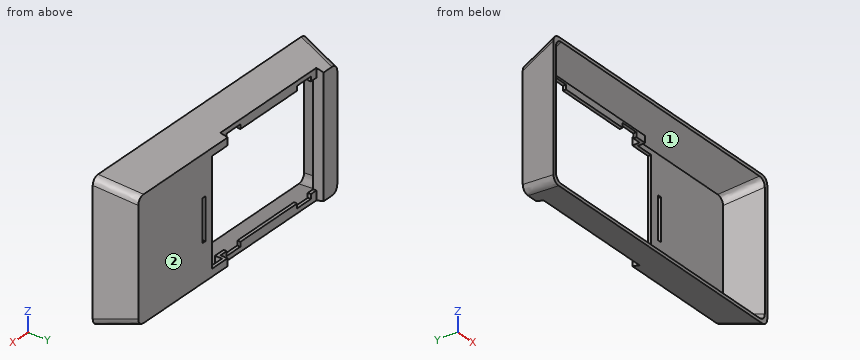
```python
from build123d import *

# Parameters (mm, degrees)
CUT_EXTRUDE1_REACH             = 225.719
SKETCH4_W                      = 175
SKETCH4_H                      = 10
CUT_EXTRUDE1_DIRECTION_2_REACH = 225.719
SHELL1_T                       = -4.4
CUT_EXTRUDE2_DEPTH             = 224.718573366
FILLET1_R                      = 10
SKETCH7_W                      = 5.5
SKETCH7_H                      = 58
CUT_EXTRUDE4_DEPTH             = 10


with BuildPart() as part:
    # Sketch2 → Loft1 section 0
    with BuildSketch(Plane(origin=(0, 0, 0), x_dir=(1, 0, 0), z_dir=(0, 1, 0))):
        with BuildLine():
            Line((-195, 96), (195, 96))
            Line((195, 96), (195, -96))
            Line((195, -96), (-195, -96))
            Line((-195, -96), (-195, 96))
        make_face()
    # Sketch3 → Loft1 section 1
    with BuildSketch(Plane(origin=(0, 53, 0), x_dir=(1, 0, 0), z_dir=(0, 1, 0))):
        with BuildLine():
            Line((-181.5, 83), (181.5, 83))
            Line((181.5, 83), (181.5, -83))
            Line((181.5, -83), (-181.5, -83))
            Line((-181.5, -83), (-181.5, 83))
        make_face()
    loft()

    # Cut-Extrude1: up to this plane
    cut_extrude1_end = Plane(origin=(0, 22.210879785, -90.552048355), z_dir=(0, -0.23822152779764819, 0.9712108440981054))
    # Sketch4 → Cut-Extrude1 (cut, up to the surface)
    with BuildSketch(Plane.XY, mode=Mode.PRIVATE) as cut_extrude1_sk1:
        with Locations((-69, 48)):
            Rectangle(SKETCH4_W, SKETCH4_H)
    cut_extrude1_tool1 = split(extrude(cut_extrude1_sk1.sketch, amount=-CUT_EXTRUDE1_REACH, mode=Mode.PRIVATE), bisect_by=cut_extrude1_end, keep=Keep.BOTH, mode=Mode.PRIVATE)
    add(cut_extrude1_tool1.solids().sort_by_distance((-69, 48, 0))[0], mode=Mode.SUBTRACT)

    # Cut-Extrude1 direction 2: up to this plane
    cut_extrude1_direction_2_end = Plane(origin=(0, 22.210879785, 90.552048355), z_dir=(0, -0.23822152779764863, -0.9712108440981052))
    # Sketch4 → Cut-Extrude1 direction 2 (cut, up to the surface)
    with BuildSketch(Plane.XY, mode=Mode.PRIVATE) as cut_extrude1_direction_2_sk1:
        with Locations((-69, 48)):
            Rectangle(SKETCH4_W, SKETCH4_H)
    cut_extrude1_direction_2_tool1 = split(extrude(cut_extrude1_direction_2_sk1.sketch, amount=CUT_EXTRUDE1_DIRECTION_2_REACH, mode=Mode.PRIVATE), bisect_by=cut_extrude1_direction_2_end, keep=Keep.BOTH, mode=Mode.PRIVATE)
    add(cut_extrude1_direction_2_tool1.solids().sort_by_distance((-69, 48, 0))[0], mode=Mode.SUBTRACT)

    # Shell1
    shell1_openings = [part.faces().sort_by_distance(p)[0] for p in [
        (0, 0, 0),
    ]]
    offset(amount=SHELL1_T, openings=shell1_openings, kind=Kind.INTERSECTION)

    # Sketch5 → Cut-Extrude2 (cut, through all)
    with BuildSketch(Plane(origin=(0, 53, 0), x_dir=(1, 0, 0), z_dir=(0, 1, 0))):
        Polygon((47, -72.7), (47, 72.7), (7, 72.7), (7, 79), (-18, 79), (-18, 72.7), (-121.5, 72.7), (-121.5, 79), (-146.5, 79), (-146.5, 72.7), (-156.5, 72.7), (-156.5, -72.7), (-146.5, -72.7), (-146.5, -79), (-121.5, -79), (-121.5, -72.7), (-18, -72.7), (-18, -79), (7, -79), (7, -72.7), align=None)
    extrude(amount=-CUT_EXTRUDE2_DEPTH, mode=Mode.SUBTRACT)

    # Fillet1
    fillet1_edges = [part.edges().sort_by_distance(p)[0] for p in [
        (-188.25, 26.5, 89.5),
        (-188.25, 26.5, -89.5),
        (188.25, 26.5, 89.5),
        (188.25, 26.5, -89.5),
        (-184.269882767, 24.3, -85.509195467),
        (-184.269882767, 24.3, 85.509195467),
        (184.269882767, 24.3, 85.509195467),
        (184.269882767, 24.3, -85.509195467),
    ]]
    fillet(fillet1_edges, radius=FILLET1_R)

    # Sketch7 → Cut-Extrude4 (cut)
    with BuildSketch(Plane(origin=(0, 53, 0), x_dir=(1, 0, 0), z_dir=(0, 1, 0))):
        with Locations((61.95, 2.369883227)):
            Rectangle(SKETCH7_W, SKETCH7_H)
    extrude(amount=-CUT_EXTRUDE4_DEPTH, mode=Mode.SUBTRACT)


solid = part.part
```
Verification items for the finished model (mm, model axes). Face numbers are marked on the shaded views. Round coordinates to 2 decimals unless told otherwise and drop trailing zeros. Put each result on its own line as item: value. Start each with the question number.
(1) Material ranges on line 1 along Z through (x, y) = (-11, 3); line 2 along Z through (x, y) = (108, 5); line 3 along Y through (x, z) = (129, 62.5), recorded low to high.
(2) Depth check by flat-ended pin: pin 1 Ø16 at (x, y) = (29.5, 47) entering from -Z; pin 2 Ø10 at (y, z) = (6, 52.5) entering from -X; pin 3 Ø3 at (y, z) = (30, -19) entering from +X. Enter the tip coordinate at first touch or a pass-through.
(3) Section check A-A (z = -16.5). State how many separate pieces and enclosed holes the cut face has, then the cut area to 3 significant figures.
(4) Draft check along Z on the marked faces 1 and 2. Enter one of: +Z half, -Z half, draft (parallel to the pull), parting line (faces both ways), or undercut.
Completed:
1. line 1: z = -95.26 to -90.73, 90.73 to 95.26
1. line 2: z = -94.77 to -90.24, 90.24 to 94.77
1. line 3: y = 48.6 to 53
2. pin 1: stops at z = -86.43
2. pin 2: stops at x = -194.75
2. pin 3: stops at x = 187.74
3. separate pieces: 3
3. enclosed holes: 0
3. area: 1,170 mm2
4. face 1: undercut
4. face 2: draft
